Job drawing, mm, ordinate dimensions from the low corner. One solid piece. A direction names the side the tool comes from. Round coordinates to 2 decimals unless told otherwise and drop trailing zeros. Order: outer loops, then holes, each group sorted by start corner. A loop starts at its lowest first (then second) coordinate and runs counter-clockwise, first axis right, second up. Notation, with made-up numbers: M 86.25,-36.75 L 142.25,-36.75 A20 cw 142.25,-29.75 Z; hole C 35.25,16 d3. An arc over 180 degrees is marked long. Answer as a JSON object with one key per item and string values. Group by question number.
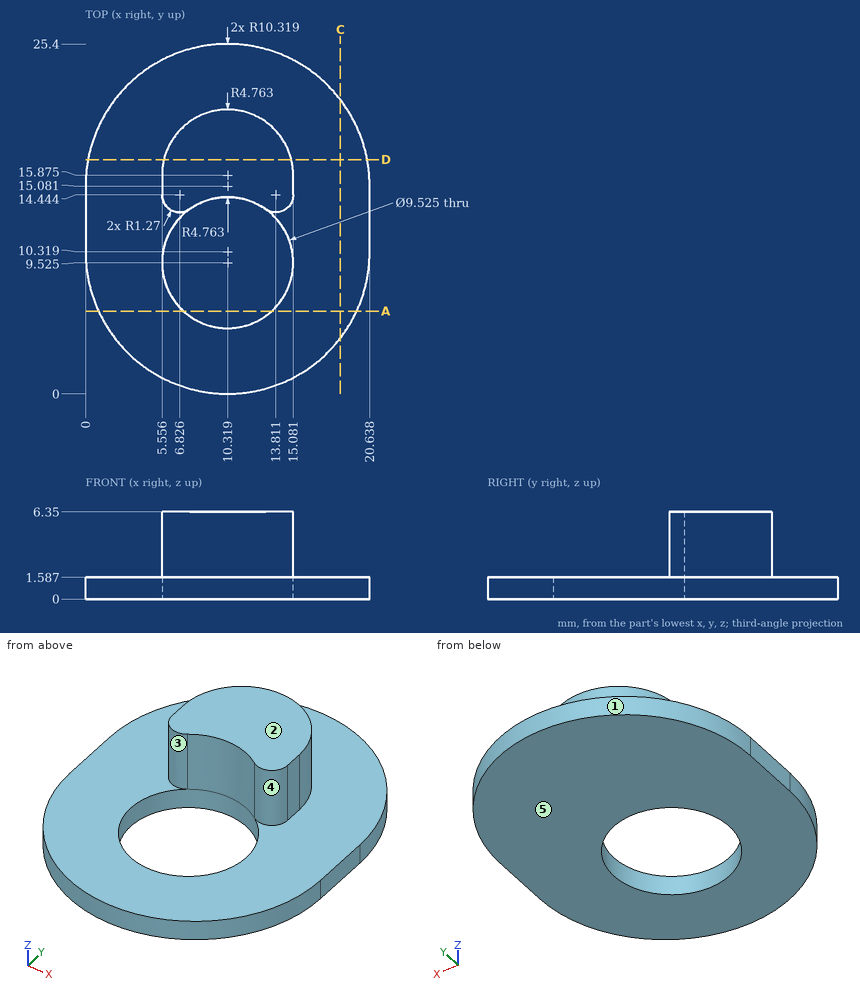
Item 1: 3-axis set-ups, long thin cutter, end or side, ignore diameter. For the marked faces 4 and 5: which of +Z, -Z, +X, -X, +Y, -Y reach the whole face in a straight line?
Item 2: Two-plate mould, pull along X, no slides. Class the marked faces 1, 2 and 3: +X half, -X half, draft (parallel to the pull), parting line (faces both ways), or undercut.
Item 3: Cut at A-A, the plane y = 6. Give the cut face in (x, z), and give its area (3 significant figures).
Item 4: Drill centre lines: line 1 (Z direction, x = 7.25, y = 24); line 2 (X direction, y = 15, z = 2.25); line 3 (Y direction, x = 9.25, z = 1) (1 decimal). Where is each one in solid material? Low to high. Write a range as [from, to].
Item 5: Cut at D-D, the plane y = 17. Give the cut face in (x, z).
Item 6: Flat gauge pins, fed straight in: pin 1 Ø0.7 at (y, z) = (15.5, 3.5) entering from -X; pin 2 Ø1.6 at (y, z) = (15, 4.5) entering from +X; pin 3 Ø3 at (x, z) = (12, 5) entering from +Y. Where does each tip first touch, or does it go through?
Item 7: Cut at C-C, the plane x = 18.5. Give the cut face in (y, z).
Response values:
{
 "1": {"face 4": "+Z, -Y", "face 5": "-Z, +X, -X, +Y, -Y"},
 "2": {"face 1": "parting line", "face 2": "draft", "face 3": "undercut"},
 "3": {"outline": "M 0.95,0 L 7.12,0 L 7.12,1.59 L 0.95,1.59 Z; M 13.52,0 L 19.69,0 L 19.69,1.59 L 13.52,1.59 Z", "area": "19.6 mm^2"},
 "4": {"line 1": "[0, 1.59]", "line 2": "[5.56, 15.08]", "line 3": "[0.1, 4.9], [14.2, 25.3]"},
 "5": {"outline": "M 0.18,0 L 20.46,0 L 20.46,1.59 L 14.95,1.59 L 14.95,6.35 L 5.69,6.35 L 5.69,1.59 L 0.18,1.59 Z"},
 "6": {"pin 1": "x = 5.56", "pin 2": "x = 15.08", "pin 3": "y = 20.63"},
 "7": {"outline": "M 4.03,0 L 21.37,0 L 21.37,1.59 L 4.03,1.59 Z"}
}
